Work out the finished part from the listing and answer in its coordinate system (mm). Round coordinates to 2 decimals unless told otherwise and drop trailing zeros. Order: outer loops, then holes, each group sorted by start corner. A loop starts at its lowest first (then second) coordinate and runs counter-clockwise, first axis right, second up. Notation, with made-up numbers: M 54,65 L 94,65 A23 cw 94,94 Z; hole C -5.75,-37 d2. An arc over 180 degrees is marked long. Answer as a JSON object with one key per item and string values. Group by question number.
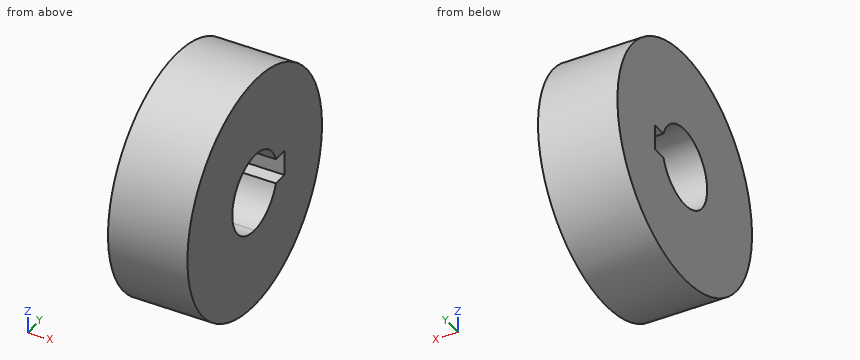
from build123d import *

# Parameters (mm, degrees)
SKETCH1_R           = 15
BOSS_EXTRUDE1_DEPTH = 10


with BuildPart() as part:
    # Sketch1 → Boss-Extrude1 (new body)
    with BuildSketch(Plane(origin=(0, 0, 0), x_dir=(0, 0, -1), z_dir=(1, 0, 0))):
        Circle(SKETCH1_R)
        with BuildLine():
            Line((1.615081939, 6.6), (1.615081939, 4.731966857))
            ThreePointArc((1.615081939, 4.731966857), (4.0666577, 2.909002433), (5, 0))
            ThreePointArc((5, 0), (-2.909002433, -4.0666577), (-1.615081939, 4.731966857))
            Line((-1.615081939, 4.731966857), (-1.615081939, 6.6))
            Line((-1.615081939, 6.6), (1.615081939, 6.6))
        make_face(mode=Mode.SUBTRACT)
    extrude(amount=BOSS_EXTRUDE1_DEPTH)


solid = part.part
Item 1: Find section A-A (z = 0). Give the vertices of the cut face in (x, y).
Item 2: Find section D-D (z = 7). Give the vertices of the cut face in (x, y).
Item 3: Consider L1, parallel to Y at x = 5.25, z = 0; L2, parallel to Y at x = 4.25, z = -3; L3, parallel to Z at x = 9.75, y = 3.75. Determine where each line is inside the solid, lowest interval first.
Item 4: Find section B-B (y = 4.25). Give the vertices of the cut face in (x, z).
Item 5: Find section C-C (x = 7.25). Give the vertices of the cut face in (y, z), and give its area (3 significant figures).
Item 6: Each of these flat-tipped pins is pushed along its axis until it touches: pin 1 (5 mm diameter, centred on x = 2.5, y = -4, fed in from -Z); pin 2 (1 mm diameter, centred on x = 5, y = 6.5, fed in from +Z); pin 3 (0.9 mm diameter, centred on x = 3, y = 6, fed in from -Z); pin 4 (6 mm diameter, centred on y = 0, z = 0, fed in from +X). Where does it stop, or does it pass through?
Responses:
{
 "1": {"outline": "M 0,-15 L 10,-15 L 10,-5 L 0,-5 Z; M 0,6.6 L 10,6.6 L 10,15 L 0,15 Z"},
 "2": {"outline": "M 0,-13.27 L 10,-13.27 L 10,13.27 L 0,13.27 Z"},
 "3": {"L1": "y = -15 to -5, 6.6 to 15", "L2": "y = -14.7 to -4, 4 to 14.7", "L3": "z = -14.52 to -3.31, 3.31 to 14.52"},
 "4": {"outline": "M 0,-14.39 L 10,-14.39 L 10,-2.63 L 0,-2.63 Z; M 0,2.63 L 10,2.63 L 10,14.39 L 0,14.39 Z"},
 "5": {"outline": "C 0,0 d30; hole M 4.73,-1.62 L 6.6,-1.62 L 6.6,1.62 L 4.73,1.62 A5 ccw long Z", "area": "623 mm^2"},
 "6": {"pin 1": "stops at z = -14.92", "pin 2": "stops at z = 13.75", "pin 3": "stops at z = -13.94", "pin 4": "passes through"}
}
